```python
from build123d import *

# Parameters (mm, degrees)
SKETCH2_W           = 21
SKETCH2_H           = 30
BOSS_EXTRUDE1_DEPTH = 7
SKETCH3_W           = 12
SKETCH3_H           = 28
CUT_EXTRUDE1_DEPTH  = 4.5
SKETCH4_W           = 4.231229846
SKETCH4_H           = 28
CUT_EXTRUDE2_DEPTH  = 6.5
SKETCH8_W           = 7.5
SKETCH8_H           = 3.5
BOSS_EXTRUDE3_DEPTH = 17.5
SKETCH10_R          = 0.95
CUT_EXTRUDE4_DEPTH  = 3
SKETCH11_W          = 1.35
SKETCH11_H          = 3.5
SKETCH11_W_2        = 1.65
CUT_EXTRUDE5_DEPTH  = 17.5
SKETCH7_W           = 2.2
SKETCH7_H           = 4
SKETCH7_W_2         = 2.4
CUT_EXTRUDE6_DEPTH  = 2
SKETCH13_W          = 14.768770154
SKETCH13_H          = 15.6
CUT_EXTRUDE8_DEPTH  = 2.5
SKETCH14_W          = 7.585503546
SKETCH14_H          = 28.388252519
CUT_EXTRUDE9_DEPTH  = 10
SKETCH15_W          = 30
SKETCH15_H          = 34.4
BOSS_EXTRUDE4_DEPTH = 1.5
SKETCH16_W          = 13
SKETCH16_H          = 16
SKETCH16_W_2        = 17.5
SKETCH16_H_2        = 4.2
SKETCH16_W_3        = 10.4
SKETCH16_H_3        = 12
CUT_EXTRUDE10_DEPTH = 2
SKETCH17_R          = 1
SKETCH17_R_2        = 1.5
CUT_EXTRUDE11_DEPTH = 2
SKETCH18_W          = 1.5
SKETCH18_H          = 30
BOSS_EXTRUDE5_DEPTH = 12
SKETCH19_R          = 3
CUT_EXTRUDE12_DEPTH = 10


with BuildPart() as part:
    # Sketch2 → Boss-Extrude1 (new body)
    with BuildSketch(Plane.XY):
        Rectangle(SKETCH2_W, SKETCH2_H)
    extrude(amount=BOSS_EXTRUDE1_DEPTH)

    # Sketch3 → Cut-Extrude1 (cut)
    with BuildSketch(Plane.XY.offset(7)):
        with Locations((3.5, 0)):
            Rectangle(SKETCH3_W, SKETCH3_H)
    extrude(amount=-CUT_EXTRUDE1_DEPTH, mode=Mode.SUBTRACT)

    # Sketch4 → Cut-Extrude2 (cut)
    with BuildSketch(Plane(origin=(0, 0, 0), x_dir=(-1, 0, 0), z_dir=(0, 0, -1))):
        with Locations((7.384385077, 0)):
            Rectangle(SKETCH4_W, SKETCH4_H)
    extrude(amount=-CUT_EXTRUDE2_DEPTH, mode=Mode.SUBTRACT)

    # Sketch8 → Boss-Extrude3 (add)
    with BuildSketch(Plane(origin=(0, 0, 0), x_dir=(-1, 0, 0), z_dir=(0, 0, -1))):
        with Locations((0.75, 10.55)):
            Rectangle(SKETCH8_W, SKETCH8_H)
        with Locations((0.75, -10.55)):
            Rectangle(SKETCH8_W, SKETCH8_H)
    extrude(amount=BOSS_EXTRUDE3_DEPTH)

    # Sketch10 → Cut-Extrude4 (cut)
    with BuildSketch(Plane(origin=(0, 0, -17.5), x_dir=(-1, 0, 0), z_dir=(0, 0, -1))):
        with Locations((0.9, 10.55)):
            Circle(SKETCH10_R)
        with Locations(Location((0.9, -10.55, 0), (0, 0, 180))):
            Circle(SKETCH10_R)
    extrude(amount=-CUT_EXTRUDE4_DEPTH, mode=Mode.SUBTRACT)

    # Sketch11 → Cut-Extrude5 (cut)
    with BuildSketch(Plane(origin=(0, 0, -17.5), x_dir=(-1, 0, 0), z_dir=(0, 0, -1))):
        with Locations((3.825, -10.55)):
            Rectangle(SKETCH11_W, SKETCH11_H)
        with Locations((-2.175, -10.55)):
            Rectangle(SKETCH11_W_2, SKETCH11_H)
        with Locations((3.825, 10.55)):
            Rectangle(SKETCH11_W, SKETCH11_H)
        with Locations((-2.175, 10.55)):
            Rectangle(SKETCH11_W_2, SKETCH11_H)
    extrude(amount=-CUT_EXTRUDE5_DEPTH, mode=Mode.SUBTRACT)

    # Sketch7 → Cut-Extrude6 (cut)
    with BuildSketch(Plane.XY.offset(7)):
        with Locations((-7.5, 11)):
            Rectangle(SKETCH7_W, SKETCH7_H)
        with Locations((-7.4, -11)):
            Rectangle(SKETCH7_W_2, SKETCH7_H)
    extrude(amount=-CUT_EXTRUDE6_DEPTH, mode=Mode.SUBTRACT)

    # Sketch13 → Cut-Extrude8 (cut)
    with BuildSketch(Plane(origin=(0, 0, 0), x_dir=(-1, 0, 0), z_dir=(0, 0, -1))):
        with Locations((-2.115614923, 0)):
            Rectangle(SKETCH13_W, SKETCH13_H)
    extrude(amount=-CUT_EXTRUDE8_DEPTH, mode=Mode.SUBTRACT)

    # Sketch14 → Cut-Extrude9 (cut)
    with BuildSketch(Plane(origin=(0, 0, 0), x_dir=(-1, 0, 0), z_dir=(0, 0, -1))):
        with Locations((-5.707248227, -0.19412626)):
            Rectangle(SKETCH14_W, SKETCH14_H)
    extrude(amount=-CUT_EXTRUDE9_DEPTH, mode=Mode.SUBTRACT)

    # Sketch15 → Boss-Extrude4 (add)
    with BuildSketch(Plane(origin=(0, 0, -17.5), x_dir=(-1, 0, 0), z_dir=(0, 0, -1))):
        with Locations((-11.85, 0)):
            Rectangle(SKETCH15_W, SKETCH15_H)
    extrude(amount=BOSS_EXTRUDE4_DEPTH)

    # Sketch16 → Cut-Extrude10 (cut)
    with BuildSketch(Plane(origin=(0, 0, -19), x_dir=(-1, 0, 0), z_dir=(0, 0, -1))):
        with Locations((-3.35, 0)):
            Rectangle(SKETCH16_W, SKETCH16_H)
        with Locations((-5.6, -15.1)):
            Rectangle(SKETCH16_W_2, SKETCH16_H_2)
        with Locations((-5.6, 15.1)):
            Rectangle(SKETCH16_W_2, SKETCH16_H_2)
        with Locations((-21.65, 0)):
            Rectangle(SKETCH16_W_3, SKETCH16_H_3)
    extrude(amount=-CUT_EXTRUDE10_DEPTH, mode=Mode.SUBTRACT)

    # Sketch17 → Cut-Extrude11 (cut)
    with BuildSketch(Plane(origin=(0, 0, -19), x_dir=(-1, 0, 0), z_dir=(0, 0, -1))):
        with Locations((-22.55, -15.875)):
            Circle(SKETCH17_R)
        with Locations((-24.85, -11.5)):
            Circle(SKETCH17_R_2)
        with Locations((-22.55, 15.875)):
            Circle(SKETCH17_R)
        with Locations((-24.85, 11.5)):
            Circle(SKETCH17_R_2)
    extrude(amount=-CUT_EXTRUDE11_DEPTH, mode=Mode.SUBTRACT)

    # Sketch18 → Boss-Extrude5 (add)
    with BuildSketch(Plane.ZY.offset(10.5)):
        with Locations((6.25, 0)):
            Rectangle(SKETCH18_W, SKETCH18_H)
    extrude(amount=BOSS_EXTRUDE5_DEPTH)

    # Sketch19 → Cut-Extrude12 (cut)
    with BuildSketch(Plane(origin=(0, 0, 5.5), x_dir=(-1, 0, 0), z_dir=(0, 0, -1))):
        with Locations(Location((18.589045846, 5.243756264, 0), (0, 0, 90))):
            Circle(SKETCH19_R)
        with Locations(Location((18.589045846, -5.243756264, 0), (0, 0, 90))):
            Circle(SKETCH19_R)
    extrude(amount=-CUT_EXTRUDE12_DEPTH, mode=Mode.SUBTRACT)


solid = part.part
```
Input: part model. Units: mm. Frame: model coordinates. A direction names the side the tool comes from. Give positions to 0.01 mm unless a question says otherwise; leave off trailing zeros. Order: outer loops, then holes, each group sorted by start corner. A loop starts at its lowest first (then second) coordinate and runs counter-clockwise, first axis right, second up. Notation, with made-up numbers: M 49.5,22 L 107.5,22 A22 ccw 107.5,60 Z; hole C 77.25,26.5 d8. An arc over 180 degrees is marked long. One line per question, with ' | ' between items.
1) Section A-A on x = 24.85. Output: boundary loops of the cut face in (y, z).
Filled in:
outline: M -17.2,-19 L -13,-19 L -13,-17.5 L -17.2,-17.5 Z; M -10,-19 L -6,-19 L -6,-17.5 L -10,-17.5 Z; M 6,-19 L 10,-19 L 10,-17.5 L 6,-17.5 Z; M 13,-19 L 17.2,-19 L 17.2,-17.5 L 13,-17.5 Z
2) Section B-B on z = -8.5. Output: boundary loops of the cut face in (x, y), and give its area (3 significant figures).
Filled in:
outline: M -3.15,-12.3 L 1.35,-12.3 L 1.35,-8.8 L -3.15,-8.8 Z; M -3.15,8.8 L 1.35,8.8 L 1.35,12.3 L -3.15,12.3 Z | area: 31.5 mm2
3) Section C-C on y = -10.55. State how many separate pieces and enclosed holes the cut face has, and give its area (3 significant figures).
Filled in:
separate pieces: 4 | enclosed holes: 1 | area: 178 mm2
4) Access query for faces 4 (the face through (-3.15, -11, -9)), 5 (the face through (1.914, -12, 2)), 6 (the face through (-2, 7.8, 1)). Directions: +Z, -Z, +X, -X, +Y, -Y. A direction counts if a zero-diameter tool reaches every point of the face in a straight line with its end or side. Return the directions, or none.
Filled in:
face 4: -Z, -X, +Y, -Y | face 5: +Z | face 6: -Z
5) Draft query along Y for faces 1 (the face through (-16, 0, 5.5)), 2 (the face through (-2, 15, 3)), 3 (the face through (-2, -7.8, 1)). Return one class per face: pulls with the +Y half, pulls with the -Y half, needs draft (parallel to the pull), parting line crosses it, or undercut.
Filled in:
face 1: needs draft | face 2: pulls with the +Y half | face 3: undercut
6) Contact query for flat-ended pins moving along their axis: P1, Ø8, axis at y = -9, z = -2.5, coming from the +X side; P2, Ø3, axis at x = -1, z = 1.5, coming from the -Y side; P3, Ø2, axis at x = -7.5, z = 2.5, coming from the +Y side; P4, Ø1.8, axis at x = 24.85, y = -11.5, coming from the -Z side. Output: stop coordinate, or through.
Filled in:
P1: stops at x = 10.5 | P2: stops at y = -15 | P3: stops at y = 15 | P4: passes through
7) Ray query, L1, parallel to X at y = 11, z = 2.75; L2, parallel to Y at x = 24.85, z = -18.05; L3, parallel to Y at x = 22.55, z = -18.6 (3 decimals). Return the intervals inside material, ascending.
Filled in:
L1: x = -10.5 to -9.5, -5.27 to -2.5, 9.5 to 10.5 | L2: y = -17.2 to -13, -10 to -6, 6 to 10, 13 to 17.2 | L3: y = -17.2 to -16.875, -14.875 to -6, 6 to 14.875, 16.875 to 17.2
